For this review, take the finished solid that the model builds, in its own axes (mm). Coordinates: 2 decimals unless noted, no trailing zeros. Loops run counter-clockwise (first coordinate to the right, second up) from the corner with the lowest first, then second, coordinate; pieces in that order, holes last. Notation, with made-up numbers: (49.5, 55) -> (55.5, 55) arc R22 ccw to (55.5, 85) -> close; hole circle Ø4 at (62, 66). An arc over 180 degrees is marked (long way). Use a Markdown table: item, result.
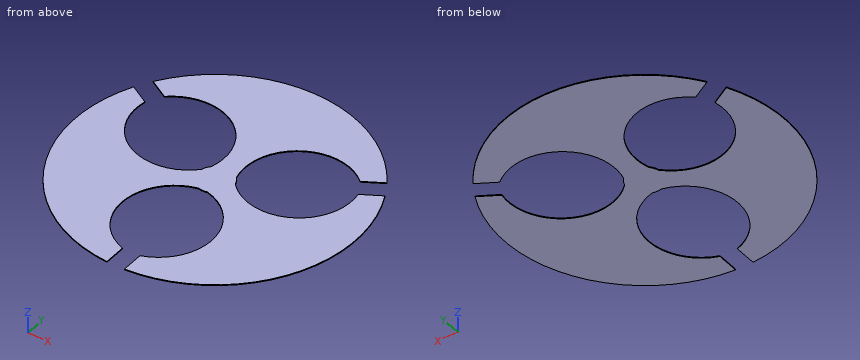
from build123d import *

# Parameters (mm, degrees)
F1_DEPTH = 1


with BuildPart() as f1:
    # F0 (on Top) → F1 (new body)
    with BuildSketch(Plane.XY):
        with BuildLine():
            ThreePointArc((-10, -134.687194), (-51.059593, -75.137453), (-5, -19.364917))
            ThreePointArc((-5, -19.364917), (0, -20), (5, -19.364917))
            ThreePointArc((5, -19.364917), (51.059593, -75.137453), (10, -134.687194))
            Line((10, -134.687194), (10, -159.687194))
            ThreePointArc((10, -159.687194), (138.564065, -80), (143.293167, 71.183343))
            Line((143.293167, 71.183343), (121.642532, 58.683343))
            ThreePointArc((121.642532, 58.683343), (90.60074, -6.650179), (19.27051, 5.352331))
            ThreePointArc((19.27051, 5.352331), (17.320508, 10), (14.27051, 14.012585))
            ThreePointArc((14.27051, 14.012585), (39.541146, 81.787631), (111.642532, 76.003851))
            Line((111.642532, 76.003851), (133.293167, 88.503851))
            ThreePointArc((133.293167, 88.503851), (0, 160), (-133.293167, 88.503851))
            Line((-133.293167, 88.503851), (-111.642532, 76.003851))
            ThreePointArc((-111.642532, 76.003851), (-39.541146, 81.787631), (-14.27051, 14.012585))
            ThreePointArc((-14.27051, 14.012585), (-17.320508, 10), (-19.27051, 5.352331))
            ThreePointArc((-19.27051, 5.352331), (-90.60074, -6.650179), (-121.642532, 58.683343))
            Line((-121.642532, 58.683343), (-143.293167, 71.183343))
            ThreePointArc((-143.293167, 71.183343), (-138.564065, -80), (-10, -159.687194))
            Line((-10, -159.687194), (-10, -134.687194))
        make_face()
    extrude(amount=F1_DEPTH)


solid = f1.part
(1) Take a section at D-D on x = -75. Write out the cut boundary in (y, z), plus the area to 3 significant figures.
Found:
| item | result |
|---|---|
| outline | (-141.33, 0) -> (-12.2, 0) -> (-12.2, 1) -> (-141.33, 1) -> close; (91.09, 0) -> (141.33, 0) -> (141.33, 1) -> (91.09, 1) -> close |
| area | 179 mm^2 |
(2) Take a section at B-B on z = 0.3. Write out the cut boundary in (x, y).
Found:
| item | result |
|---|---|
| outline | (-143.29, 71.18) arc R160 ccw to (-10, -159.69) -> (-10, -134.69) arc R60 cw to (-5, -19.36) arc R20 ccw to (5, -19.36) arc R60 cw to (10, -134.69) -> (10, -159.69) arc R160 ccw to (143.29, 71.18) -> (121.64, 58.68) arc R60 cw to (19.27, 5.35) arc R20 ccw to (14.27, 14.01) arc R60 cw to (111.64, 76) -> (133.29, 88.5) arc R160 ccw to (-133.29, 88.5) -> (-111.64, 76) arc R60 cw to (-14.27, 14.01) arc R20 ccw to (-19.27, 5.35) arc R60 cw to (-121.64, 58.68) -> close |
(3) For line 1 along X through (y, z) = (81.5, 0.1); line 2 along X through (y, z) = (79, 0.6); line 3 along Y through (x, z) = (-35, 0.2), list the stretches that pass through material, from the lowest coordinate up.
Found:
| item | result |
|---|---|
| line 1 | x = -121.16 to -104.43, -39.09 to 39.09, 104.43 to 121.16 |
| line 2 | x = -116.83 to -108, -35.53 to 35.53, 108 to 116.83 |
| line 3 | y = -156.12 to -118.65, -36.82 to -6.57, 78.59 to 156.12 |
(4) Take a section at C-C on y = 81.5. Write out the cut boundary in (x, z), plus the area to 3 significant figures.
Found:
| item | result |
|---|---|
| outline | (-121.16, 0) -> (-104.43, 0) -> (-104.43, 1) -> (-121.16, 1) -> close; (-39.09, 0) -> (39.09, 0) -> (39.09, 1) -> (-39.09, 1) -> close; (104.43, 0) -> (121.16, 0) -> (121.16, 1) -> (104.43, 1) -> close |
| area | 112 mm^2 |
(5) Take a section at A-A on y = -32. Write out the cut boundary in (x, z), plus the area to 3 significant figures.
Found:
| item | result |
|---|---|
| outline | (-156.77, 0) -> (-29.95, 0) -> (-29.95, 1) -> (-156.77, 1) -> close; (29.95, 0) -> (156.77, 0) -> (156.77, 1) -> (29.95, 1) -> close |
| area | 254 mm^2 |
